For this review, use the dimensioned drawing (mm, ordinates from the lowest corner) and the shaded views. Give positions to 0.01 mm unless a question says otherwise; leave off trailing zeros. Loops run counter-clockwise (first coordinate to the right, second up) from the corner with the lowest first, then second, coordinate; pieces in that order, holes last. Notation, with made-up numbers: (53.25, 88) -> (67.25, 88) arc R31 ccw to (67.25, 117) -> close; hole circle Ø6 at (23.25, 68). An arc over 180 degrees is marked (long way). Write each question's results on one line, items separated by ' | '. Start each with the question number.
Q1. We need section B-B (y = 167). Write out the cut boundary in (x, z), plus the area to 4 significant figures.
Q2. Wall thickness on L1, parallel to Y at x = 116.25, z = 0.85; L2, parallel to X at y = 157, z = 1; L3, parallel to X at y = 88, z = 1.75: over which ranges is each line inside the solid? List them lowest first. Write a range as [from, to].
Q3. We need section C-C (x = 116.25). Write out the cut boundary in (y, z), plus the area to 3 significant figures.
Q4. We need section A-A (x = 8). Write out the cut boundary in (y, z), plus the area to 3 significant figures.
Q5. We need section D-D (y = 78.5). Write out the cut boundary in (x, z).
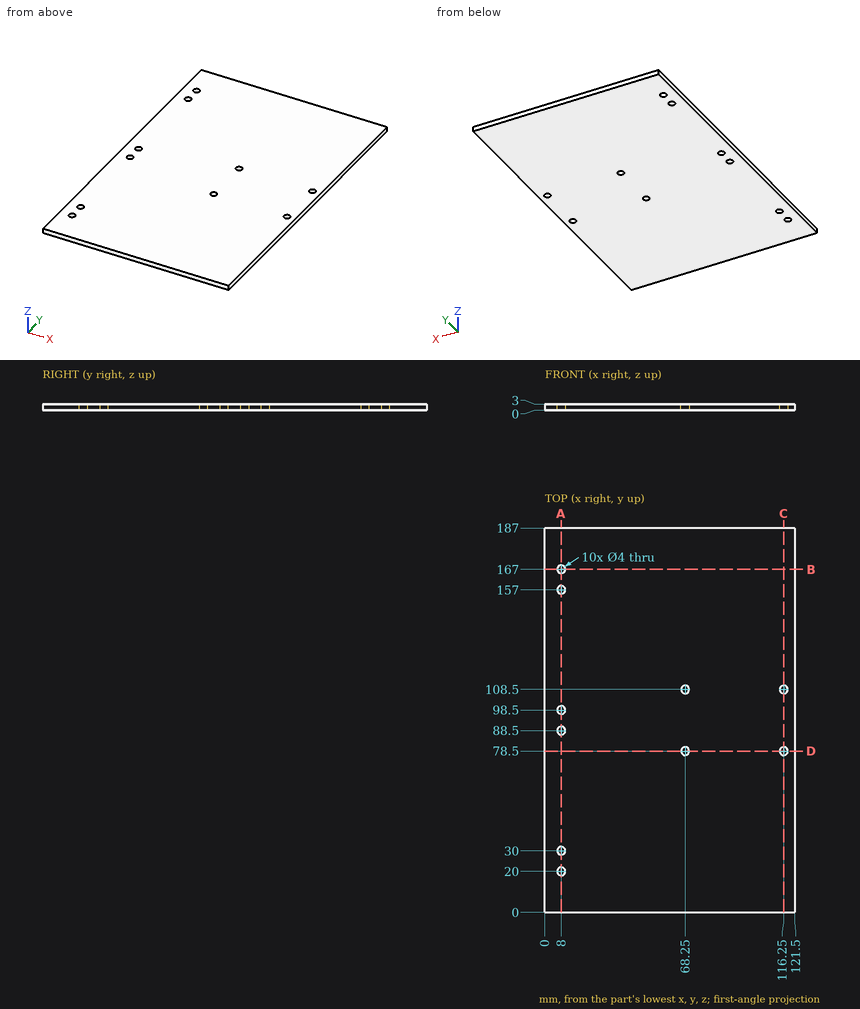
Output:
1) outline: (0, 0) -> (6, 0) -> (6, 3) -> (0, 3) -> close; (10, 0) -> (121.5, 0) -> (121.5, 3) -> (10, 3) -> close | area: 352.5 mm2
2) L1: [0, 76.5], [80.5, 106.5], [110.5, 187] | L2: [0, 6], [10, 121.5] | L3: [0, 6.06], [9.94, 121.5]
3) outline: (0, 0) -> (76.5, 0) -> (76.5, 3) -> (0, 3) -> close; (80.5, 0) -> (106.5, 0) -> (106.5, 3) -> (80.5, 3) -> close; (110.5, 0) -> (187, 0) -> (187, 3) -> (110.5, 3) -> close | area: 537 mm2
4) outline: (0, 0) -> (18, 0) -> (18, 3) -> (0, 3) -> close; (22, 0) -> (28, 0) -> (28, 3) -> (22, 3) -> close; (32, 0) -> (86.5, 0) -> (86.5, 3) -> (32, 3) -> close; (90.5, 0) -> (96.5, 0) -> (96.5, 3) -> (90.5, 3) -> close; (100.5, 0) -> (155, 0) -> (155, 3) -> (100.5, 3) -> close; (159, 0) -> (165, 0) -> (165, 3) -> (159, 3) -> close; (169, 0) -> (187, 0) -> (187, 3) -> (169, 3) -> close | area: 489 mm2
5) outline: (0, 0) -> (66.25, 0) -> (66.25, 3) -> (0, 3) -> close; (70.25, 0) -> (114.25, 0) -> (114.25, 3) -> (70.25, 3) -> close; (118.25, 0) -> (121.5, 0) -> (121.5, 3) -> (118.25, 3) -> close
